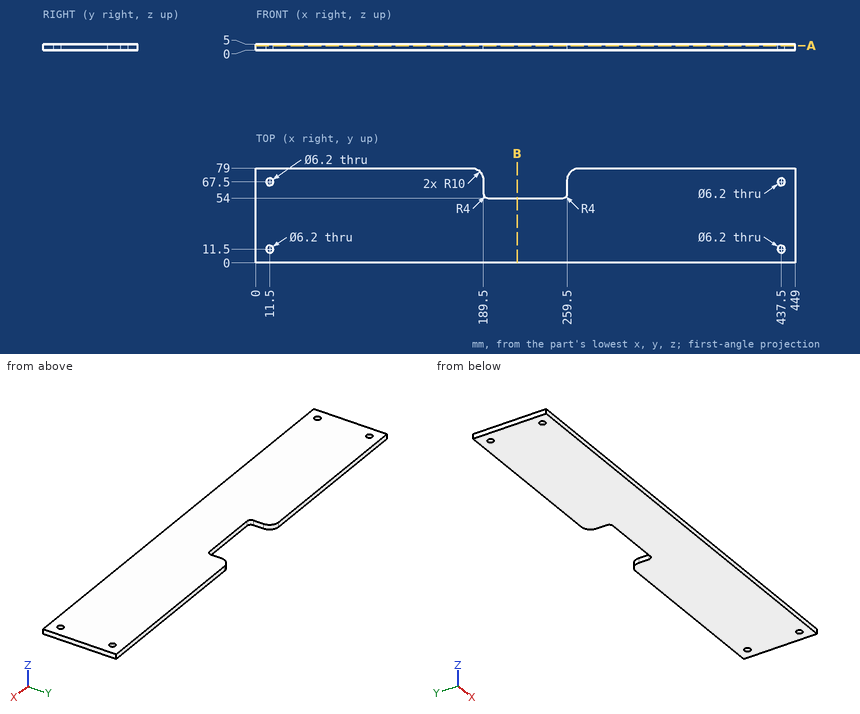
Could you check a few things on this drawing? It's one solid part, dimensions in mm from its lowest x, y, z. Give positions to 0.01 mm unless a question says otherwise; leave off trailing zeros. Write each loop counter-clockwise with the first axis right and the second up, starting at its lowest first coordinate (ties: lowest second). Pieces come first, ordered by that corner, then holes. Notation, with made-up numbers: M 70.5,3 L 81.5,3 A13 cw 81.5,9 Z; hole C 54,87.25 d4. An arc over 180 degrees is marked long. Put each result on its own line as item: value. Start each with the question number.
Item 1: If we section it at B-B, the plane x = 217.5: Write out the boundary of the cut face in (y, z).
Item 2: Will these pins go through, and if not, where does the flat tip stop? pin 1 (1.5 mm diameter, centred on y = 63, z = 1.5, fed in from -X); pin 2 (5 mm diameter, centred on x = 437.5, y = 11.5, fed in from -Z); pin 3 (1.5 mm diameter, centred on x = 213.5, z = 2.5, fed in from +Y).
Item 3: If we section it at A-A, the plane z = 3.7: Write out the boundary of the cut face in (x, y), then the cut area to 3 significant figures.
Item 4: I need wall thicknesses on L1, parallel to Y at x = 437.5, z = 2.2; L2, parallel to X at y = 59, z = 3.65; L3, parallel to X at y = 14, z = 0.7. Which ranges of each line are inside material? Lowest first, please. Write a range as from..to.
Values:
1. outline: M 0,0 L 54,0 L 54,5 L 0,5 Z
2. pin 1: x = 0
2. pin 2: through
2. pin 3: y = 54
3. outline: M 0,0 L 449,0 L 449,79 L 269.5,79 A10 ccw 259.5,69 L 259.5,58 A4 cw 255.5,54 L 193.5,54 A4 cw 189.5,58 L 189.5,69 A10 ccw 179.5,79 L 0,79 Z; hole C 11.5,11.5 d6.2; hole C 11.5,67.5 d6.2; hole C 437.5,11.5 d6.2; hole C 437.5,67.5 d6.2
3. area: 33,600 mm²
4. L1: 0..8.4, 14.6..64.4, 70.6..79
4. L2: 0..189.5, 259.5..449
4. L3: 0..9.67, 13.33..435.67, 439.33..449
